Could you check a few things on this model? Use its own coordinates, in mm. Face numbers are marked on the shaded views. Round coordinates to 2 decimals unless told otherwise and drop trailing zeros. Order: outer loops, then holes, each group sorted by start corner. A loop starts at its lowest first (then second) coordinate and runs counter-clockwise, first axis right, second up. Notation, with made-up numbers: (20.5, 5.25) - (36.5, 5.25) arc R11 ccw to (36.5, 22.25) - close; hole circle Ø7 at (57.5, 40.25). An arc over 180 degrees is marked (long way). Use one line per item in the form item = value.
from build123d import *

# Parameters (mm, degrees)
EXTRUDE_1_DEPTH    = 5
HOLE_WIZARD_M3_1_D = 2.5


with BuildPart() as part:
    # 草圖1 → 填料-伸長1 (new body)
    with BuildSketch(Plane(origin=(0, 0, 0), x_dir=(1, 0, 0), z_dir=(0, 1, 0))):
        with BuildLine():
            ThreePointArc((-67.5, 45), (-47.72970773, -2.72970773), (0, -22.5))
            ThreePointArc((0, -22.5), (22.5, 0), (0, 22.5))
            ThreePointArc((0, 22.5), (-15.909902577, 29.090097423), (-22.5, 45))
            ThreePointArc((-22.5, 45), (-45, 22.5), (-67.5, 45))
        make_face()
    extrude(amount=-EXTRUDE_1_DEPTH)

    # M3 螺紋孔1 (through all)
    with Locations(Plane(origin=(0, 0, 0), x_dir=(1, 0, 0), z_dir=(0, 1, 0))):
        with Locations((-32.24496324, 13.611111111), (0, 0)):
            Hole(HOLE_WIZARD_M3_1_D / 2)


solid = part.part
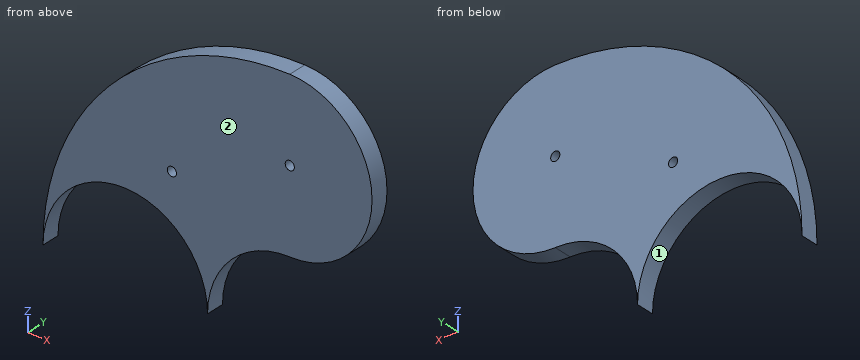
Item 1: I need wall thicknesses on L1, parallel to X at y = -1.75, z = 1; L2, parallel to Z at x = -1, y = -3.2; L3, parallel to X at y = -3.05, z = -33. Which ranges of each line are inside material? Lowest first, please.
Found:
L1 = -49.4 to -0.75, 0.75 to 22.48
L2 = -22.52 to -0.75, 0.75 to 22.49
L3 = -66.42 to -64.03, -25.97 to -19.03
Item 2: Imagine slicing it at B-B on y = -3.2. Please give me the cut outline in (x, z), plus the area to 3 significant figures.
Found:
outline = (-67.5, -45) arc R22.5 cw to (-22.5, -45) arc R22.5 cw to (0, -22.5) arc R22.5 ccw to (0, 22.5) arc R67.5 ccw to start; hole circle Ø2.5 at (-32.24, -13.61); hole circle Ø2.5 at (0, 0)
area = 3,170 mm2
Item 3: If we mould it in two halves opening along X, with no side actions, what happens to the marked faces 1 and 2? For each: released by +X, released by -X, zero draft, split by the parting line, or undercut.
Found:
face_1 = undercut
face_2 = zero draft
Item 4: Imagine slicing it at C-C on x = 8. Please give me the cut outline in (y, z), plus the area to 3 significant figures.
Found:
outline = (-5, -21.03) - (0, -21.03) - (0, 21.03) - (-5, 21.03) - close
area = 210 mm2
Item 5: Will this pin go through, and if not, where does the flat tip stop? P1, Ø1, axis at y = -1.5, z = -4.5, coming from the +X side.
Found:
P1 = 22.14
Item 6: Imagine slicing it at D-D on z = -16.5. Please give me the cut outline in (x, y), plus the area to 3 significant figures.
Found:
outline = (-61.19, -5) - (15.3, -5) - (15.3, 0) - (-61.19, 0) - close
area = 382 mm2
Item 7: Imagine slicing it at A-A on z = 0. Please give me the cut outline in (x, y).
Found:
outline = (-50.31, -5) - (-1.25, -5) - (-1.25, 0) - (-50.31, 0) - close; (1.25, -5) - (22.5, -5) - (22.5, 0) - (1.25, 0) - close
